The model under review builds one solid part; all positions refer to its coordinate system, in mm. A direction names the side the tool comes from. Coordinates: 2 decimals unless noted, no trailing zeros. Loops run counter-clockwise (first coordinate to the right, second up) from the corner with the lowest first, then second, coordinate; pieces in that order, holes last. Notation, with made-up numbers: M -5.5,68.5 L 43.5,68.5 A25 cw 43.5,81.5 Z; hole C 26.5,25 d8. An arc over 180 degrees is marked long. Return JSON: item names as keys, results as strings.
```python
from build123d import *

# Parameters (mm, degrees)
BASE_FLANGE1_DEPTH            = 2
EDGE_FLANGE1_DEPTH            = 125
EDGE_FLANGE2_DEPTH            = 30
EDGE_FLANGE3_STRIP_W          = 12
EDGE_FLANGE3_STRIP_H          = 2
EDGE_FLANGE3_STRIP_CUT_DEPTH  = 125
EDGE_FLANGE3_DEPTH            = 125
EDGE_FLANGE4_STRIP_W          = 12
EDGE_FLANGE4_STRIP_H          = 2
EDGE_FLANGE4_STRIP_CUT_DEPTH  = 125
EDGE_FLANGE4_DEPTH            = 125
SKETCH19_W                    = 53
SKETCH19_H                    = 271
CUT_EXTRUDE2_DEPTH            = 4
M4_CLEARANCE_HOLE1_AT_2_COUNT = 2
M4_CLEARANCE_HOLE1_AT_2_PITCH = 78.333333333
M4_CLEARANCE_HOLE1_AT_3_COUNT = 2
M4_CLEARANCE_HOLE1_AT_3_PITCH = 156.666666667
M4_CLEARANCE_HOLE1_AT_4_COUNT = 2
M4_CLEARANCE_HOLE1_AT_4_PITCH = 235
M4_CLEARANCE_HOLE2_D          = 4.8
SKETCH25_R                    = 4.5
CUT_EXTRUDE3_DEPTH            = 10
CUT_EXTRUDE4_START            = -2
SKETCH26_R                    = 4.5
CUT_EXTRUDE4_DEPTH            = 2
F_6_0_6_DIAMETER_HOLE1_D      = 6
M8_CLEARANCE_HOLE1_D          = 9
M8_CLEARANCE_HOLE1_DEPTH      = 2
FILLET3_R                     = 3
M8_CLEARANCE_HOLE2_D          = 9
EDGE_FLANGE5_DEPTH            = 82.996938457
F_7_0_7_DIAMETER_HOLE1_D      = 7
F_7_0_7_DIAMETER_HOLE1_DEPTH  = 2
FILLET4_R                     = 5
EDGE_FLANGE6_DEPTH            = 285
EDGE_FLANGE6_START            = -2
EDGE_FLANGE6_FLAT_DEPTH       = 2
FILLET5_R                     = 1
FILLET6_R                     = 3


# Sheet-metal steps are written as plain solids
with BuildPart() as part:
    # Sketch1 → Base-Flange1 (new body)
    with BuildSketch(Plane.XY):
        with BuildLine():
            Line((15, 0), (-15, 0))
            Line((-15, 0), (-15, 65))
            Line((-15, 65), (110, 65))
            Line((110, 65), (110, 29))
            Line((110, 29), (20, 29))
            ThreePointArc((20, 29), (16.464466094, 27.535533906), (15, 24))
            Line((15, 24), (15, 0))
        make_face()
    extrude(amount=-BASE_FLANGE1_DEPTH)

    # Edge-Flange1 section (across the edge) → Edge-Flange1 (add)
    with BuildSketch(Plane(origin=(-15, 67, -2), x_dir=(0, -1, 0), z_dir=(1, 0, 0))):
        with BuildLine():
            Line((-2, 2), (-2, 289))
            Line((-2, 289), (0, 289))
            Line((0, 289), (0, 2))
            ThreePointArc((0, 2), (0.585786438, 0.585786438), (2, 0))
            Line((2, 0), (2, -2))
            ThreePointArc((2, -2), (-0.828427125, -0.828427125), (-2, 2))
        make_face()
    extrude(amount=EDGE_FLANGE1_DEPTH)

    # Edge-Flange2 section (across the edge) → Edge-Flange2 (add)
    with BuildSketch(Plane(origin=(15, -2, -2), x_dir=(0, 1, 0), z_dir=(-1, 0, 0))):
        with BuildLine():
            Line((-2, 2), (-2, 30))
            Line((-2, 30), (0, 30))
            Line((0, 30), (0, 2))
            ThreePointArc((0, 2), (0.585786438, 0.585786438), (2, 0))
            Line((2, 0), (2, -2))
            ThreePointArc((2, -2), (-0.828427125, -0.828427125), (-2, 2))
        make_face()
    extrude(amount=EDGE_FLANGE2_DEPTH)

    # Edge-Flange3 strip (across the edge) → Edge-Flange3 strip cut (cut)
    with BuildSketch(Plane(origin=(-15, 67, -291), x_dir=(0, 0, 1), z_dir=(1, 0, 0))):
        with Locations((-4, -1)):
            Rectangle(EDGE_FLANGE3_STRIP_W, EDGE_FLANGE3_STRIP_H)
    extrude(amount=EDGE_FLANGE3_STRIP_CUT_DEPTH, mode=Mode.SUBTRACT)

    # Edge-Flange3 section (across the edge) → Edge-Flange3 (add)
    with BuildSketch(Plane(origin=(-15, 67, -291), x_dir=(0, 0, 1), z_dir=(1, 0, 0))):
        with BuildLine():
            Line((-2, 2), (-2, 69))
            Line((-2, 69), (0, 69))
            Line((0, 69), (0, 2))
            ThreePointArc((0, 2), (0.585786438, 0.585786438), (2, 0))
            Line((2, 0), (2, -2))
            ThreePointArc((2, -2), (-0.828427125, -0.828427125), (-2, 2))
        make_face()
    extrude(amount=EDGE_FLANGE3_DEPTH)

    # Edge-Flange4 strip (across the edge) → Edge-Flange4 strip cut (cut)
    with BuildSketch(Plane(origin=(110, -2, -293), x_dir=(0, 1, 0), z_dir=(-1, 0, 0))):
        with Locations((-4, -1)):
            Rectangle(EDGE_FLANGE4_STRIP_W, EDGE_FLANGE4_STRIP_H)
    extrude(amount=EDGE_FLANGE4_STRIP_CUT_DEPTH, mode=Mode.SUBTRACT)

    # Edge-Flange4 section (across the edge) → Edge-Flange4 (add)
    with BuildSketch(Plane(origin=(110, -2, -293), x_dir=(0, 1, 0), z_dir=(-1, 0, 0))):
        with BuildLine():
            Line((-2, 2), (-2, 30.8))
            Line((-2, 30.8), (0, 30.8))
            Line((0, 30.8), (0, 2))
            ThreePointArc((0, 2), (0.585786438, 0.585786438), (2, 0))
            Line((2, 0), (2, -2))
            ThreePointArc((2, -2), (-0.828427125, -0.828427125), (-2, 2))
        make_face()
    extrude(amount=EDGE_FLANGE4_DEPTH)

    # Sketch19 → Cut-Extrude2 (cut)
    with BuildSketch(Plane(origin=(0, 69, 0), x_dir=(1, 0, 0), z_dir=(0, 1, 0))):
        with Locations((68.5, 146.5)):
            Rectangle(SKETCH19_W, SKETCH19_H)
    extrude(amount=-CUT_EXTRUDE2_DEPTH, mode=Mode.SUBTRACT)

    # Sketch22 → M4 Clearance Hole1 (revolve, cut)
    with BuildSketch(Plane(origin=(102.041079456, 69, -264), x_dir=(0, 0, 1), z_dir=(1, 0, 0))):
        Polygon((0, 0), (0, 5.351936393), (2.25, 4), (2.25, 0), align=None)
    m4_clearance_hole1 = revolve(axis=Axis((102.041079456, 75.35, -264), (0, -1, 0)), mode=Mode.SUBTRACT)

    # M4 Clearance Hole1 at 2: M4 Clearance Hole1 ×2
    with Locations(*[(0, 0, i * M4_CLEARANCE_HOLE1_AT_2_PITCH) for i in range(1, M4_CLEARANCE_HOLE1_AT_2_COUNT)]):
        add(m4_clearance_hole1, mode=Mode.SUBTRACT)

    # M4 Clearance Hole1 at 3: M4 Clearance Hole1 ×2
    with Locations(*[(0, 0, i * M4_CLEARANCE_HOLE1_AT_3_PITCH) for i in range(1, M4_CLEARANCE_HOLE1_AT_3_COUNT)]):
        add(m4_clearance_hole1, mode=Mode.SUBTRACT)

    # M4 Clearance Hole1 at 4: M4 Clearance Hole1 ×2
    with Locations(*[(0, 0, i * M4_CLEARANCE_HOLE1_AT_4_PITCH) for i in range(1, M4_CLEARANCE_HOLE1_AT_4_COUNT)]):
        add(m4_clearance_hole1, mode=Mode.SUBTRACT)

    # M4 Clearance Hole2 (through all)
    with Locations(Plane(origin=(0, 69, 0), x_dir=(1, 0, 0), z_dir=(0, 1, 0))):
        with Locations((103.2, 217.4925), (103.2, 75.4925), (32.3, 217.4925), (32.3, 75.4925)):
            Hole(M4_CLEARANCE_HOLE2_D / 2)

    # Mirror1: M4 Clearance Hole1 across plane
    add(m4_clearance_hole1.mirror(Plane.ZY.offset(-68.5)), mode=Mode.SUBTRACT)

    # Mirror1 copy 1 sketch → Mirror1 copy 1 (revolve, cut)
    with BuildSketch(Plane(origin=(34.958920544, 69, -185.666666667), x_dir=(0, 0, 1), z_dir=(-1, 0, 0))):
        Polygon((0, 0), (0, -5.351936393), (2.25, -4), (2.25, 0), align=None)
    revolve(axis=Axis((34.958920544, 75.35, -185.666666667), (0, 1, 0)), mode=Mode.SUBTRACT)

    # Mirror1 copy 2 sketch → Mirror1 copy 2 (revolve, cut)
    with BuildSketch(Plane(origin=(34.958920544, 69, -107.333333333), x_dir=(0, 0, 1), z_dir=(-1, 0, 0))):
        Polygon((0, 0), (0, -5.351936393), (2.25, -4), (2.25, 0), align=None)
    revolve(axis=Axis((34.958920544, 75.35, -107.333333333), (0, 1, 0)), mode=Mode.SUBTRACT)

    # Mirror1 copy 3 sketch → Mirror1 copy 3 (revolve, cut)
    with BuildSketch(Plane(origin=(34.958920544, 69, -29), x_dir=(0, 0, 1), z_dir=(-1, 0, 0))):
        Polygon((0, 0), (0, -5.351936393), (2.25, -4), (2.25, 0), align=None)
    revolve(axis=Axis((34.958920544, 75.35, -29), (0, 1, 0)), mode=Mode.SUBTRACT)

    # Sketch25 → Cut-Extrude3 (cut)
    with BuildSketch(Plane(origin=(0, 0, -2), x_dir=(-1, 0, 0), z_dir=(0, 0, -1))):
        with BuildLine():
            ThreePointArc((-80.541079456, 44), (-85.041079456, 39.5), (-89.541079456, 44))
            Line((-89.541079456, 44), (-89.541079456, 29))
            Line((-89.541079456, 29), (-80.541079456, 29))
            Line((-80.541079456, 29), (-80.541079456, 44))
        make_face()
        with Locations((-85.041079456, 44)):
            Circle(SKETCH25_R)
        with Locations((-52.041079456, 44)):
            Circle(SKETCH25_R)
        with BuildLine():
            Line((-56.541079456, 44), (-56.541079456, 29))
            Line((-56.541079456, 29), (-47.541079456, 29))
            Line((-47.541079456, 29), (-47.541079456, 44))
            ThreePointArc((-47.541079456, 44), (-52.041079456, 39.5), (-56.541079456, 44))
        make_face()
    extrude(amount=-CUT_EXTRUDE3_DEPTH, mode=Mode.SUBTRACT)

    # Sketch26 → Cut-Extrude4 (cut)
    with BuildSketch(Plane.XY.offset(-291).offset(CUT_EXTRUDE4_START)):
        with Locations((85.041079456, 44)):
            Circle(SKETCH26_R)
        with Locations((52.041079456, 44)):
            Circle(SKETCH26_R)
    extrude(amount=CUT_EXTRUDE4_DEPTH, mode=Mode.SUBTRACT)

    # Ø6.0 (6) Diameter Hole1 (through all)
    with Locations(Plane.XY):
        with Locations((99.738017913, 34.5), (70.344140999, 53.5), (66.738017913, 34.5), (37.344140999, 53.5)):
            Hole(F_6_0_6_DIAMETER_HOLE1_D / 2)

    # M8 Clearance Hole1
    with Locations(Plane(origin=(0, -2, 0), x_dir=(1, 0, 0), z_dir=(0, 1, 0))):
        with Locations((0, 18)):
            Hole(M8_CLEARANCE_HOLE1_D / 2, depth=M8_CLEARANCE_HOLE1_DEPTH)

    # Fillet3
    fillet3_edges = [part.edges().sort_by_distance(p)[0] for p in [
        (15, -3, -32),
        (-15, -3, -32),
    ]]
    fillet(fillet3_edges, radius=FILLET3_R)

    # M8 Clearance Hole2 (through all)
    with Locations(Plane(origin=(0, -2, 0), x_dir=(1, 0, 0), z_dir=(0, 1, 0))):
        with Locations((85, 309.4), (10, 309.4)):
            Hole(M8_CLEARANCE_HOLE2_D / 2)

    # Edge-Flange5 section (across the edge) → Edge-Flange5 (add)
    with BuildSketch(Plane(origin=(110, -2, -325.8), x_dir=(0, 0, 1), z_dir=(-1, 0, 0))):
        with BuildLine():
            Line((-2, 2), (-2, 20))
            Line((-2, 20), (0, 20))
            Line((0, 20), (0, 2))
            ThreePointArc((0, 2), (0.585786438, 0.585786438), (2, 0))
            Line((2, 0), (2, -2))
            ThreePointArc((2, -2), (-0.828427125, -0.828427125), (-2, 2))
        make_face()
    extrude(amount=EDGE_FLANGE5_DEPTH)

    # Ø7.0 (7) Diameter Hole1
    with Locations(Plane.XY.offset(-325.8)):
        with Locations((90, 9), (47.003061543, 9)):
            Hole(F_7_0_7_DIAMETER_HOLE1_D / 2, depth=F_7_0_7_DIAMETER_HOLE1_DEPTH)

    # Fillet4
    fillet4_edges = [part.edges().sort_by_distance(p)[0] for p in [
        (110, 18, -326.8),
        (27.003061543, 18, -326.8),
    ]]
    fillet(fillet4_edges, radius=FILLET4_R)

    # Edge-Flange6 bend section (across the edge) → Edge-Flange6 (add)
    with BuildSketch(Plane(origin=(112, 67, -289), x_dir=(-1, 0, 0), z_dir=(0, 0, 1))):
        with BuildLine():
            Line((-2, 2), (0, 2))
            ThreePointArc((0, 2), (0.585786438, 0.585786438), (2, 0))
            Line((2, 0), (2, -2))
            ThreePointArc((2, -2), (-0.828427125, -0.828427125), (-2, 2))
        make_face()
    extrude(amount=EDGE_FLANGE6_DEPTH)

    # Edge-Flange6 profile (on flange) → Edge-Flange6 flat (add)
    with BuildSketch(Plane(origin=(112, 67, 0), x_dir=(0, 0, -1), z_dir=(-1, 0, 0)).offset(EDGE_FLANGE6_START)):
        Polygon((4, 2), (289, 2), (289, 3), (293, 3), (293, 37.882021368), (291.992065684, 37.882021368), (1.007934316, 37.882021368), (0, 37.882021368), (0, 3), (4, 3), align=None)
    extrude(amount=EDGE_FLANGE6_FLAT_DEPTH)

    # Fillet5
    fillet5_edges = [part.edges().sort_by_distance(p)[0] for p in [
        (110, 29, -1),
        (113, 29.117978632, 0),
        (113, 29.117978632, -293),
    ]]
    fillet(fillet5_edges, radius=FILLET5_R)

    # Fillet6
    fillet6_edges = [part.edges().sort_by_distance(p)[0] for p in [
        (-15, -3, -323.8),
    ]]
    fillet(fillet6_edges, radius=FILLET6_R)


solid = part.part
```
1. Add section D-D on z = -18. Give the boundary of the cut face in (x, y), plus the area to 3 significant figures.
Check values:
{"outline": "M -15,-4 L -4.5,-4 L -4.5,-2 L -15,-2 Z; M -15,67 L 42,67 L 42,69 L -15,69 Z; M 4.5,-4 L 15,-4 L 15,-2 L 4.5,-2 Z; M 95,67 L 110,67 A2 cw 112,65 L 112,29.12 L 114,29.12 L 114,65 A4 ccw 110,69 L 95,69 Z", "area": "267 mm²"}
2. The part is to be moulded in two halves that separate along Y. For faces 5 (the face through (114, 47, -144)), 6 (the face through (48, -2, -310)), 7 (the face through (63.877, 35.401, -292.014)), say which applies: released by +Y, released by -Y, zero draft, split by the parting line, or undercut.
Check values:
{"face 5": "zero draft", "face 6": "released by +Y", "face 7": "undercut"}
3. To check wall thickness, follow line 1 (X direction, y = 34, z = -1); line 2 (Z direction, x = 68, y = 0); line 3 (Z direction, x = 20, y = 41). State the ranges of each line that lie inside material, in increasing order.
Check values:
{"line 1": "-15 to 47.54, 56.54 to 63.78, 69.7 to 80.54, 89.54 to 96.78, 102.7 to 110, 112 to 114", "line 2": "-327.8 to -325.8, -293 to -291", "line 3": "-293 to -291, -2 to 0"}
4. Machinability: for faces 1 (the face through (0.59, -3.01, -22.46)), 2 (the face through (4, -2, -21)), 3 (the face through (10.59, -3.01, -313.86)), 4 (the face through (47, 33, -293)), which of the approach directions +Z, -Z, +X, -X, +Y, -Y give a long, thin tool a straight path to every point of the face, cutting with its end or side? Answer none if there is none.
Check values:
{"face 1": "-Y", "face 2": "+X, -X", "face 3": "+Y, -Y", "face 4": "+X, -X, +Y"}
5. Add section C-C on y = 60. Give the boundary of the cut face in (x, z).
Check values:
{"outline": "M -15,-293 L 110,-293 L 110,-291 L -15,-291 Z; M -15,-2 L 110,-2 L 110,0 L -15,0 Z; M 112,-293 L 114,-293 L 114,0 L 112,0 Z"}
6. Add section A-A on z = -57. Give the boundary of the cut face in (x, y), plus the area to 3 significant figures.
Check values:
{"outline": "M -15,67 L 42,67 L 42,69 L -15,69 Z; M 95,67 L 110,67 A2 cw 112,65 L 112,29.12 L 114,29.12 L 114,65 A4 ccw 110,69 L 95,69 Z", "area": "225 mm²"}
7. Add section B-B on x = 0. Give the boundary of the cut face in (y, z), plus the area to 3 significant figures.
Check values:
{"outline": "M -4,-323.8 L -2,-323.8 L -2,-295 A2 cw 0,-293 L 65,-293 A4 ccw 69,-289 L 69,-4 A4 ccw 65,0 L 0,0 A4 ccw -4,-4 L -4,-13.5 L -2,-13.5 L -2,-4 A2 cw 0,-2 L 65,-2 A2 cw 67,-4 L 67,-289 A2 cw 65,-291 L 0,-291 A4 ccw -4,-295 Z; M -4,-32 L -2,-32 L -2,-22.5 L -4,-22.5 Z", "area": "963 mm²"}
8. Insertion check: pin 1 Ø14.5 at (x, z) = (68, -305) entering from +Y; pin 2 Ø1.5 at (x, z) = (33, -210) entering from -Y; pin 3 Ø4 at (x, y) = (74, 10.5) entering from +Z. Each pin has a flat end and moves straight along its axis. Give the tip position at first contact, or say it passes through.
Check values:
{"pin 1": "y = -2", "pin 2": "y = 67", "pin 3": "z = -291"}
